Verification items for the finished model (mm, model axes). A direction names the side the tool comes from. Round coordinates to 2 decimals unless told otherwise and drop trailing zeros. Write each loop counter-clockwise with the first axis right and the second up, starting at its lowest first coordinate (ties: lowest second). Pieces come first, ordered by that corner, then holes. Notation, with made-up numbers: M 44,-33 L 90,-33 A8 cw 90,-23 Z; hole C -30,73.25 d8. An arc over 180 degrees is marked long. Write each question's results on one line, items separated by ' | '.
Solid Edge part; units mm, degrees
sketch "Sketch1" plane through (0, 0, 0) normal (0, 0, 1) x (1, 0, 0)
  line L0 (-96.1079, -46.8841) -> (3.8921, -46.8841)
  line L1 (3.8921, -46.8841) -> (3.8921, 53.1159)
  line L2 (3.8921, 53.1159) -> (-96.1079, 53.1159)
  line L3 (-96.1079, 53.1159) -> (-96.1079, -46.8841)
  dimension "D1" = 96.1079
  dimension "D2" = 3.8921
extrude "Protrusion1" add sketch "Sketch1" along normal blind 75
sketch "Sketch2" plane through (-96.1079, 3.1159, 2.5) normal (-1, 0, 0) x (0, 1, 0)
  circle A0 centre (-40, -80) radius 5
  line L0 (32.5, -87.5) -> (47.5, -87.5)
  line L1 (47.5, -87.5) -> (47.5, -72.5)
  line L2 (47.5, -72.5) -> (32.5, -72.5)
  line L3 (32.5, -72.5) -> (32.5, -87.5)
  circle A1 centre (40, -80) radius 5
  line L4 (-47.5, -87.5) -> (-32.5, -87.5)
  line L5 (-32.5, -87.5) -> (-32.5, -72.5)
  line L6 (-32.5, -72.5) -> (-47.5, -72.5)
  line L7 (-47.5, -72.5) -> (-47.5, -87.5)
  dimension "D1" = 47.5
  dimension "D2" = 47.5
  dimension "D3" = 32.5
  dimension "D4" = 47.5
extrude "ExtrudedProtrusion_2" add sketch "Sketch2" against normal blind 10
mirror "Mirror1" about plane through (-46.1079, 0, 0) normal (1, 0, 0) of "ExtrudedProtrusion_2"
sketch "Sketch3" plane through (-96.1079, 3.1159, 10) normal (-1, 0, 0) x (0, -1, 0)
  line L0 (-5, -10) -> (5, -10)
  line L1 (5, -10) -> (5, -8)
  line L2 (5, -8) -> (-5, -8)
  line L3 (-5, -8) -> (-5, -10)
  dimension "D1" = 5
  dimension "D2" = 5
extrude "Cutout1" cut sketch "Sketch3" against normal through all
1) Sectioned sample at A-A, the plane z = 82.5. Count the separate pieces of the cut face and the enclosed holes in it, and give its area (3 significant figures).
Calculated:
separate pieces: 8 | enclosed holes: 0 | area: 200 mm²
2) Depth check by flat-ended pin: P1, Ø16, axis at y = 43.12, z = 82.5, coming from the +X side; P2, Ø7.5, axis at y = -36, z = 82.5, coming from the +X side; P3, Ø8, axis at x = 0, z = 79.5, coming from the -Y side; P4, Ø8, axis at x = -89, z = 79.5, coming from the +Y side. Enter the tip coordinate at first touch or a pass-through.
Calculated:
P1: stops at x = 3.89 | P2: passes through | P3: stops at y = -44.38 | P4: stops at y = 50.62
3) Draft check along Z on faces 5 (the cylindrical face through (-91.178, 45.423, 86.936)), 6 (the flat face through (-47, -46.884, 37)), 7 (the flat face through (-47, 31, 0)). Enter one of: pulls with the +Z half, pulls with the -Z half, needs draft (parallel to the pull), parting line crosses it, or undercut.
Calculated:
face 5: undercut | face 6: needs draft | face 7: pulls with the -Z half
4) Sectioned sample at C-C, the plane y = -14.5. Record the cut outline in (x, z), and give its area (3 significant figures).
Calculated:
outline: M -96.11,0 L 3.89,0 L 3.89,75 L -96.11,75 Z | area: 7,500 mm²
5) Material ranges on line 1 (Y direction, x = 0.5, z = 82.5); line 2 (X direction, y = 48.5, z = 80); line 3 (Z direction, x = -81, y = 7.5), recorded low to high. Write a range as [from, to].
Calculated:
line 1: y = [-44.38, -41.88], [-31.88, -29.38], [35.62, 38.12], [48.12, 50.62] | line 2: x = [-96.11, -86.11], [-6.11, 3.89] | line 3: z = [2, 75]
6) Access from +Z, -Z, +X, -X, +Y, -Y to the whole of each face (thin tool, end or side, straight path). Record for faces 1 (the flat face through (-91, -44.384, 82)), 2 (the flat face through (-1, -29.384, 82)), 3 (the flat face through (-47, 3, 2)), 4 (the flat face through (-6.108, 43, 77)).
Calculated:
face 1: +Z, +X, -X, -Y | face 2: +Z, +X, -X | face 3: -Z, +X, -X | face 4: +Z, +Y, -Y
7) Sectioned sample at B-B, the plane x = -16. Record the cut outline in (y, z).
Calculated:
outline: M -46.88,0 L -1.88,0 L -1.88,2 L 8.12,2 L 8.12,0 L 53.12,0 L 53.12,75 L -46.88,75 Z
